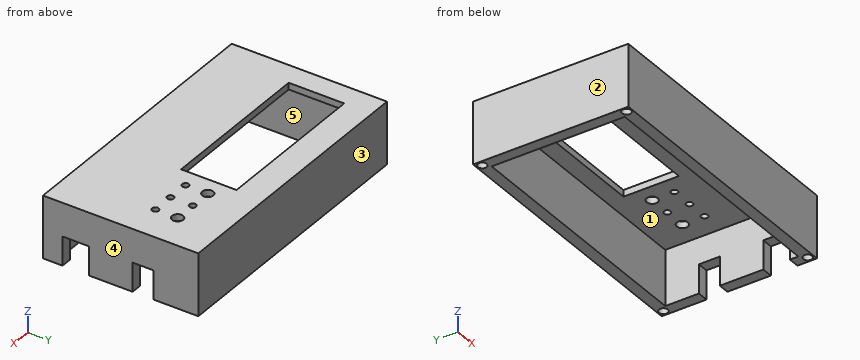
```python
from build123d import *

# Parameters (mm, degrees)
SKETCH1_W           = 125
SKETCH1_H           = 70
BOSS_EXTRUDE1_DEPTH = 3
SKETCH2_W           = 71.3
SKETCH2_H           = 25
CUT_EXTRUDE1_DEPTH  = 5
SKETCH4_R           = 2.5
SKETCH4_R_2         = 1.5
CUT_EXTRUDE2_DEPTH  = 5
SKETCH5_W           = 125
SKETCH5_H           = 70
SKETCH5_W_2         = 115
SKETCH5_H_2         = 60
BOSS_EXTRUDE2_DEPTH = 25
SKETCH6_R           = 2
CUT_EXTRUDE3_DEPTH  = 10
SKETCH7_W           = 13
SKETCH7_H           = 12
SKETCH7_H_2         = 9.422573881
CUT_EXTRUDE4_DEPTH  = 10


with BuildPart() as part:
    # Sketch1 → Boss-Extrude1 (new body)
    with BuildSketch(Plane.XY):
        with Locations((62.5, 35)):
            Rectangle(SKETCH1_W, SKETCH1_H)
    extrude(amount=BOSS_EXTRUDE1_DEPTH)

    # Sketch2 → Cut-Extrude1 (cut)
    with BuildSketch(Plane.XY.offset(3)):
        with Locations((45.65, 45)):
            Rectangle(SKETCH2_W, SKETCH2_H)
    extrude(amount=-CUT_EXTRUDE1_DEPTH, mode=Mode.SUBTRACT)

    # Sketch4 → Cut-Extrude2 (cut)
    with BuildSketch(Plane.XY.offset(3)):
        with Locations((89.3, 50)):
            Circle(SKETCH4_R)
        with Locations((99.3, 50)):
            Circle(SKETCH4_R_2)
        with Locations((109.3, 50)):
            Circle(SKETCH4_R)
        with Locations((89.3, 40)):
            Circle(SKETCH4_R_2)
        with Locations((99.3, 40)):
            Circle(SKETCH4_R_2)
        with Locations((109.3, 40)):
            Circle(SKETCH4_R_2)
    extrude(amount=-CUT_EXTRUDE2_DEPTH, mode=Mode.SUBTRACT)

    # Sketch5 → Boss-Extrude2 (add)
    with BuildSketch(Plane(origin=(0, 0, 0), x_dir=(-1, 0, 0), z_dir=(0, 0, -1))):
        with Locations((-62.5, 35)):
            Rectangle(SKETCH5_W, SKETCH5_H)
        with Locations((-62.5, 35)):
            Rectangle(SKETCH5_W_2, SKETCH5_H_2, mode=Mode.SUBTRACT)
    extrude(amount=BOSS_EXTRUDE2_DEPTH)

    # Sketch6 → Cut-Extrude3 (cut)
    with BuildSketch(Plane(origin=(0, 0, -25), x_dir=(-1, 0, 0), z_dir=(0, 0, -1))):
        with Locations((-122.5, 67.5)):
            Circle(SKETCH6_R)
        with Locations((-2.5, 67.5)):
            Circle(SKETCH6_R)
        with Locations((-2.5, 2.5)):
            Circle(SKETCH6_R)
        with Locations((-122.5, 2.5)):
            Circle(SKETCH6_R)
    extrude(amount=-CUT_EXTRUDE3_DEPTH, mode=Mode.SUBTRACT)

    # Sketch7 → Cut-Extrude4 (cut)
    with BuildSketch(Plane(origin=(125, 0, 0), x_dir=(0, 0, -1), z_dir=(1, 0, 0))):
        with Locations((18.5, 14.8)):
            Rectangle(SKETCH7_W, SKETCH7_H)
        with Locations((18.5, 45.111286941)):
            Rectangle(SKETCH7_W, SKETCH7_H_2)
    extrude(amount=-CUT_EXTRUDE4_DEPTH, mode=Mode.SUBTRACT)


solid = part.part
```
The listing builds one solid part. Answer for the finished solid, in the listing's coordinates (mm). Face numbers are marked on the shaded views. A direction names the side the tool comes from. Give positions to 0.01 mm unless a question says otherwise; leave off trailing zeros. Order: outer loops, then holes, each group sorted by start corner. A loop starts at its lowest first (then second) coordinate and runs counter-clockwise, first axis right, second up.
1) Given P1, Ø5.5, axis at x = 121.5, y = 46.5, coming from the -Z side; P2, Ø2, axis at x = 100, y = 22.5, coming from the -Z side, each flat-ended and moving along its own axis, determine where each tip first touches the part or whether it passes through.
Reported:
P1: stops at z = -12
P2: stops at z = 0
2) Find section C-C on x = 73.5. Write down the section's boundary in (y, z).
Reported:
outline: (0, -25) - (5, -25) - (5, 0) - (32.5, 0) - (32.5, 3) - (0, 3) - close; (57.5, 0) - (65, 0) - (65, -25) - (70, -25) - (70, 3) - (57.5, 3) - close
3) Find section B-B on x = 109.3. Write down the section's boundary in (y, z), then the cut area to 3 significant figures.
Reported:
outline: (0, -25) - (5, -25) - (5, 0) - (38.5, 0) - (38.5, 3) - (0, 3) - close; (41.5, 0) - (47.5, 0) - (47.5, 3) - (41.5, 3) - close; (52.5, 0) - (65, 0) - (65, -25) - (70, -25) - (70, 3) - (52.5, 3) - close
area: 436 mm2
4) For the marked faces 4 and 5, determine the directions among +Z, -Z, +X, -X, +Y, -Y from which every point of the face is accessible in a straight line to the end or side of a thin tool.
Reported:
face 4: +Z, -Z, +X, +Y, -Y
face 5: -Z
5) Consider line 1 along Y through (x, z) = (99.3, 1.25); line 2 along Y through (x, z) = (109.3, 2.1); line 3 along Y through (x, z) = (122.5, -19.5). Determine where each line is inside the solid, lowest interval first.
Reported:
line 1: y = 0 to 38.5, 41.5 to 48.5, 51.5 to 70
line 2: y = 0 to 38.5, 41.5 to 47.5, 52.5 to 70
line 3: y = 0 to 0.5, 4.5 to 8.8, 20.8 to 40.4, 49.82 to 65.5, 69.5 to 70
6) Find section A-A on z = -16.25. Write down the section's boundary in (x, y), then the cut area to 3 significant figures.
Reported:
outline: (0, 0) - (125, 0) - (125, 8.8) - (120, 8.8) - (120, 5) - (5, 5) - (5, 65) - (120, 65) - (120, 49.82) - (125, 49.82) - (125, 70) - (0, 70) - close; (120, 20.8) - (125, 20.8) - (125, 40.4) - (120, 40.4) - close; hole circle Ø4 at (2.5, 2.5); hole circle Ø4 at (2.5, 67.5); hole circle Ø4 at (122.5, 2.5); hole circle Ø4 at (122.5, 67.5)
area: 1,690 mm2
7) Find section D-D on y = 7. Write down the section's boundary in (x, z), then the cut area to 3 significant figures.
Reported:
outline: (0, -25) - (5, -25) - (5, 0) - (120, 0) - (120, -25) - (125, -25) - (125, 3) - (0, 3) - close
area: 625 mm2
8) Determine the mould class of the marked faces 1, 2 and 3 for opening direction Y: pulls with the +Y half, pulls with the -Y half, needs draft (parallel to the pull), parting line crosses it, or undercut.
Reported:
face 1: undercut
face 2: needs draft
face 3: pulls with the +Y half
